Model file for the job. Use its own axes, mm. Face numbers are marked on the shaded views. Coordinates: 2 decimals unless noted, no trailing zeros. Order: outer loops, then holes, each group sorted by start corner. A loop starts at its lowest first (then second) coordinate and runs counter-clockwise, first axis right, second up. Notation, with made-up numbers: (77, 77.25) -> (93, 77.25) arc R26 cw to (93, 108.25) -> close; hole circle Ø8 at (8, -36). An arc over 180 degrees is marked (long way). Use CSV: the item, a comma, the result in double quotes. Start each with the question number.
(1) Pull direction Z, two halves, no side cores. Call the marked faces 1, 2 and 3: pulls with the +Z half, pulls with the -Z half, needs draft (parallel to the pull), parting line crosses it, or undercut.
(2) Cut at A-A on x = 0. Give the number of separate pieces and of enclosed holes in the cut face, plus the area to 3 significant figures.
(3) Probe L1, parallel to X at y = 8.5, z = 0 (3 decimals); L2, parallel to Y at x = 3.5, z = -13; L3, parallel to Z at x = 1.5, y = 17. List the from-to ranges inside material, lowest first.
(4) Cut at C-C on x = -14. Write the cut outline in (y, z), plus the area to 3 significant figures.
(5) Cut at D-D on z = -7. Write the cut outline in (x, y), plus the area to 3 significant figures.
(6) Pin check, flat tips, straight feed: pin 1 Ø10 at (y, z) = (25, 1.5) entering from -X (3 decimals); pin 2 Ø7.5 at (x, z) = (12.37, 7.14) entering from -Y; pin 3 Ø10 at (x, y) = (-8.5, 23) entering from +Z. Stop position of each tip, or through.
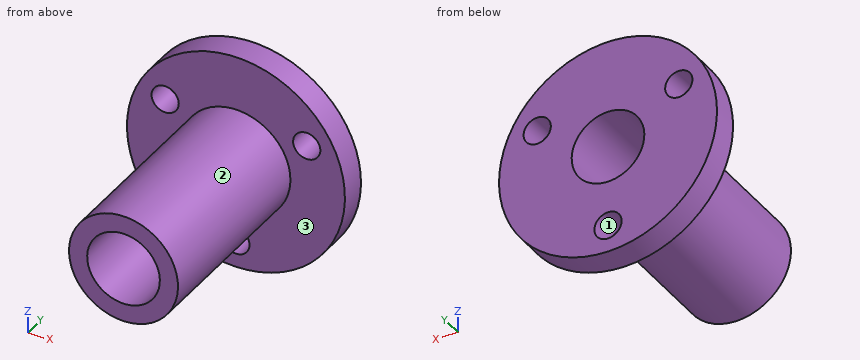
```python
from build123d import *

# Parameters (mm, degrees)
SKETCH1_R           = 19.05
BOSS_EXTRUDE1_DEPTH = 38.1
SKETCH2_R           = 19.05
SKETCH2_R_2         = 9.525
CUT_EXTRUDE1_DEPTH  = 33.3375
SKETCH3_R           = 6.35
SKETCH3_R_2         = 2.38125
CUT_EXTRUDE2_DEPTH  = 38.1


with BuildPart() as part:
    # Sketch1 → Boss-Extrude1 (new body)
    with BuildSketch(Plane(origin=(0, 0, 0), x_dir=(1, 0, 0), z_dir=(0, 1, 0))):
        with Locations(Location((0, 0, 0), (0, 0, 90))):
            Circle(SKETCH1_R)
    extrude(amount=BOSS_EXTRUDE1_DEPTH)

    # Sketch2 → Cut-Extrude1 (cut)
    with BuildSketch(Plane.XZ):
        with Locations(Location((0, 0, 0), (0, 0, 270))):
            Circle(SKETCH2_R)
        with Locations(Location((0, 0, 0), (0, 0, 270))):
            Circle(SKETCH2_R_2, mode=Mode.SUBTRACT)
    extrude(amount=-CUT_EXTRUDE1_DEPTH, mode=Mode.SUBTRACT)

    # Sketch3 → Cut-Extrude2 (cut)
    with BuildSketch(Plane(origin=(0, 38.1, 0), x_dir=(1, 0, 0), z_dir=(0, 1, 0))):
        with Locations(Location((0, 0, 0), (0, 0, 270))):
            Circle(SKETCH3_R)
        with Locations(Location((0, 14.2875, 0), (0, 0, 270))):
            Circle(SKETCH3_R_2)
        with Locations(Location((12.373337957, -7.14375, 0), (0, 0, 270))):
            Circle(SKETCH3_R_2)
        with Locations(Location((-12.373337957, -7.14375, 0), (0, 0, 270))):
            Circle(SKETCH3_R_2)
    extrude(amount=-CUT_EXTRUDE2_DEPTH, mode=Mode.SUBTRACT)


solid = part.part
```
Outcome:
1,face 1,"undercut"
1,face 2,"parting line crosses it"
1,face 3,"needs draft"
2,separate pieces,"3"
2,enclosed holes,"0"
2,area,"310 mm2"
3,L1,"-9.525 to -6.35, 6.35 to 9.525"
3,L2,"33.34 to 38.1"
3,L3,"-9.41 to -6.17, 6.17 to 9.41"
4,outline,"(33.34, -12.92) -> (38.1, -12.92) -> (38.1, 5.4) -> (33.34, 5.4) -> close; (33.34, 8.88) -> (38.1, 8.88) -> (38.1, 12.92) -> (33.34, 12.92) -> close"
4,area,"106 mm2"
5,outline,"(-17.72, 33.34) -> (-6.46, 33.34) -> (-6.46, 0) -> (6.46, 0) -> (6.46, 33.34) -> (17.72, 33.34) -> (17.72, 38.1) -> (-17.72, 38.1) -> close"
5,area,"599 mm2"
6,pin 1,"x = -9.525"
6,pin 2,"y = 33.34"
6,pin 3,"z = 8.86"
